Autodesk Inventor part; units mm, degrees
ref_plane "YZ Plane" through (0, 0, 0) normal (1, 0, 0) x (0, 1, 0)
ref_plane "XZ Plane" through (0, 0, 0) normal (0, 1, 0) x (-1, 0, 0)
ref_plane "XY Plane" through (0, 0, 0) normal (0, 0, 1) x (1, 0, 0)
sketch "Náčrt1" plane through (0, 0, 0) normal (1, 0, 0) x (0, 1, 0)
  line L0 (0, 0) -> (0, -25)
  line L1 (0, -25) -> (25, -25)
  line L2 (25, -25) -> (25, -40)
  line L3 (25, -40) -> (55, -40)
  line L4 (55, -40) -> (55, -20)
  line L5 (55, -20) -> (40, -20)
  line L6 (40, -20) -> (40, 0)
  line L7 (40, 0) -> (0, 0)
  dimension "d0" = 25
  dimension "d1" = 25
  dimension "d2" = 15
  dimension "d3" = 30
  dimension "d4" = 20
  dimension "d5" = 15
  dimension "d6" = 20
extrude "Vysunutí1" add sketch "Náčrt1" along normal blind 50
sketch "Náčrt2" plane through (50, 0, 0) normal (1, 0, 0) x (0, 0, -1)
  line L0 (20, 55) -> (20, 40)
  line L1 (40, 55) -> (20, 55)
  line L2 (20, 45) -> (40, 55)
  line L3 (40, 25) -> (40, 55)
  line L4 (40, 55) -> (20, 55)
  point P0 (0, 0)
extrude "Vysunutí2" cut sketch "Náčrt2" against normal blind 15
properties part number "4"
Read the model definition and answer for the solid it produces. Units are mm, in the model's axes. A direction names the side the tool comes from. Coordinates: 2 decimals unless noted, no trailing zeros. Write each loop counter-clockwise with the first axis right and the second up, starting at its lowest first coordinate (ties: lowest second). Pieces come first, ordered by that corner, then holes. Notation, with made-up numbers: (-19, 15) -> (23, 15) arc R24 ccw to (23, 38) -> close; hole circle Ø11 at (39.5, 16). An arc over 180 degrees is marked (long way). Return JSON: item names as keys, results as strings.
1. A cutting plane is placed at C-C (x = 30). Determine the outline of the cut face in (y, z).
Found:
{"outline": "(0, -25) -> (25, -25) -> (25, -40) -> (55, -40) -> (55, -20) -> (40, -20) -> (40, 0) -> (0, 0) -> close"}
2. Determine the mould class of faces 5 (the face through (50, 27, -20)), 6 (the face through (25, 12, -25)), 7 (the face through (0, 27, -20)) for opening direction X: pulls with the +X half, pulls with the -X half, needs draft (parallel to the pull), parting line crosses it, or undercut.
Found:
{"face 5": "pulls with the +X half", "face 6": "needs draft", "face 7": "pulls with the -X half"}
3. Each of these flat-tipped pins is pushed along its axis until it touches: P1, Ø12.5, axis at x = 33.5, y = 10, coming from the -Z side; P2, Ø2, axis at x = 16, z = -26.5, coming from the -Y side; P3, Ø6, axis at x = 37, z = -7, coming from the +Y side. Where does it stop, or does it pass through?
Found:
{"P1": "z = -25", "P2": "y = 25", "P3": "y = 40"}
4. A cutting plane is placed at D-D (z = -12). Determine the outline of the cut face in (x, y).
Found:
{"outline": "(0, 0) -> (50, 0) -> (50, 40) -> (0, 40) -> close"}
5. A cutting plane is placed at B-B (z = -31.5). Determine the outline of the cut face in (x, y).
Found:
{"outline": "(0, 25) -> (50, 25) -> (50, 50.75) -> (35, 50.75) -> (35, 55) -> (0, 55) -> close"}
6. A tool of negligible diameter and unlimited length cuts with its end or side. For faces 1 (the face through (25, 40, -10)), 2 (the face through (25, 25, -32)), 3 (the face through (43, 50, -30)), 4 (the face through (25, 0, -12)), from which of +Z, -Z, +X, -X, +Y, -Y can it reach the whole face along a straight path? Write none if from no direction.
Found:
{"face 1": "+Z, +X, -X, +Y", "face 2": "-Z, +X, -X, -Y", "face 3": "+Z, +X, +Y", "face 4": "+Z, -Z, +X, -X, -Y"}
7. Find the intervals of material crossed by line 1 along Z through (x, y) = (20, 7.5); line 2 along Y through (x, z) = (28.5, -9.5); line 3 along Y through (x, z) = (33.5, -36), in increasing order. Write a range as from..to.
Found:
{"line 1": "-25..0", "line 2": "0..40", "line 3": "25..55"}
8. A cutting plane is placed at A-A (y = 49). Determine the outline of the cut face in (x, z).
Found:
{"outline": "(0, -40) -> (50, -40) -> (50, -28) -> (35, -28) -> (35, -20) -> (0, -20) -> close"}
